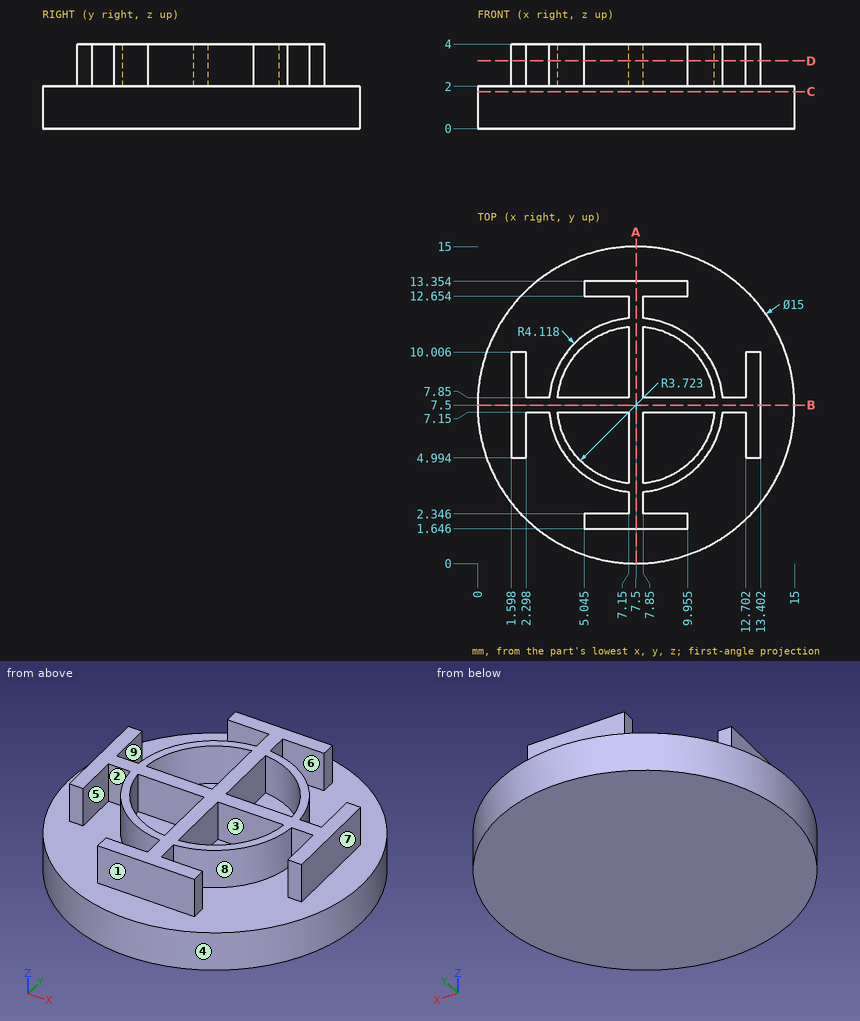
Input: dimensioned drawing with shaded views. Units: mm. Origin: part minimum x, y, z. A direction names the side the tool comes from. Round coordinates to 2 decimals unless told otherwise and drop trailing zeros. Write each loop counter-clockwise with the first axis right and the second up, starting at its lowest first coordinate (ties: lowest second). Pieces come first, ordered by that corner, then holes. Notation, with made-up numbers: (-29.5, -1.5) - (-7.5, -1.5) arc R22 cw to (-7.5, 37.5) - close; hole circle Ø2 at (85.25, 37.25). An arc over 180 degrees is marked (long way). Write item = value, one per line.
(1) Section query C-C on z = 1.75. Output: boundary loops of the cut face in (x, y).
Geometry check:
outline = circle Ø15 at (7.5, 7.5)
(2) Access query for the marked faces 5, 6, 7, 8 and 9. Directions: +Z, -Z, +X, -X, +Y, -Y. A direction counts if a zero-diameter tool reaches every point of the face in a straight line with its end or side. Return the directions, or none.
Geometry check:
face_5 = +Z, -Y
face_6 = +Z, +X
face_7 = +Z, +X, +Y, -Y
face_8 = +Z
face_9 = +Z, +Y
(3) Material intervals for probe 1 along X at (y, z) = (9.5, 2.8); probe 2 along Y at (x, z) = (7.25, 3.8); probe 3 along Z at (x, y) = (5, 2.5), sorted ascending.
Geometry check:
probe_1 = 1.6 to 2.3, 3.9 to 4.36, 7.15 to 7.85, 10.64 to 11.1, 12.7 to 13.4
probe_2 = 1.65 to 13.35
probe_3 = 0 to 2
(4) Section query D-D on z = 3.2. State how many separate pieces and enclosed holes the cut face has.
Geometry check:
separate_pieces = 1
enclosed_holes = 4
(5) Section query A-A on x = 7.5. Output: boundary loops of the cut face in (y, z).
Geometry check:
outline = (0, 0) - (15, 0) - (15, 2) - (13.35, 2) - (13.35, 4) - (1.65, 4) - (1.65, 2) - (0, 2) - close
(6) Contact query for flat-ended pins moving along their axis: pin 1 Ø0.5 at (y, z) = (3, 3) entering from -X; pin 2 Ø1 at (y, z) = (5, 3) entering from +X; pin 3 Ø0.8 at (y, z) = (2, 3) entering from +X (1 decimal). Output: stop coordinate, or through.
Geometry check:
pin_1 = 7.15
pin_2 = 13.4
pin_3 = 10
(7) Section query B-B on y = 7.5. Output: boundary loops of the cut face in (x, z), then the cut area to 3 significant figures.
Geometry check:
outline = (0, 0) - (15, 0) - (15, 2) - (13.4, 2) - (13.4, 4) - (1.6, 4) - (1.6, 2) - (0, 2) - close
area = 53.6 mm^2
(8) Pull-direction query (X, two-part tool) for the marked faces 1, 2, 3 and 4; classes: +X half, -X half, draft (parallel to the pull), parting line (faces both ways), or undercut.
Geometry check:
face_1 = draft
face_2 = undercut
face_3 = undercut
face_4 = parting line
